The listing builds one solid part. Answer for the finished solid, in the listing's coordinates (mm). Face numbers are marked on the shaded views. A direction names the side the tool comes from. Coordinates: 2 decimals unless noted, no trailing zeros. Order: outer loops, then holes, each group sorted by start corner. A loop starts at its lowest first (then second) coordinate and runs counter-clockwise, first axis right, second up. Notation, with made-up numbers: (40, 45.25) -> (55, 45.25) arc R35 cw to (55, 78.25) -> close; hole circle Ø1 at (23.25, 71.5). An arc over 180 degrees is marked (long way). Write item = value, one per line. Start each with the question number.
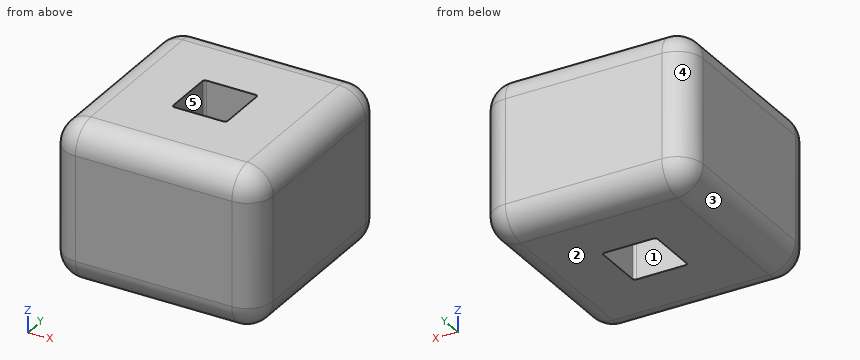
```python
from build123d import *

# Parameters (mm, degrees)
F0_W     = 400
F0_H     = 400
F0_W_2   = 104.0003
F0_H_2   = 104.0003
F1_DEPTH = 300
F2_R     = 50
F3_R     = 5


with BuildPart() as f1:
    # F0 (on Top) → F1 (new body)
    with BuildSketch(Plane.XY):
        with Locations((25.848805, -81.028401)):
            Rectangle(F0_W, F0_H)
        with Locations((25.848655, -81.028551)):
            Rectangle(F0_W_2, F0_H_2, mode=Mode.SUBTRACT)
    extrude(amount=F1_DEPTH)

    # F2
    f2_edges = [f1.edges().sort_by_distance(p)[0] for p in [
        (-174.151195, -281.028401, 150),
        (225.848805, -281.028401, 150),
        (25.848805, -281.028401, 0),
        (25.848805, -281.028401, 300),
        (225.848805, 118.971599, 150),
        (225.848805, -81.028401, 0),
        (225.848805, -81.028401, 300),
        (-174.151195, 118.971599, 150),
        (25.848805, 118.971599, 0),
        (25.848805, 118.971599, 300),
        (-174.151195, -81.028401, 0),
        (-174.151195, -81.028401, 300),
    ]]
    fillet(f2_edges, radius=F2_R)

    # F3
    f3_edges = [f1.edges().sort_by_distance(p)[0] for p in [
        (-26.151495, -29.028401, 150),
        (77.848805, -29.028401, 150),
        (77.848805, -133.028701, 150),
        (-26.151495, -133.028701, 150),
    ]]
    fillet(f3_edges, radius=F3_R)


solid = f1.part
```
Item 1: Section B-B, the plane x = 3.5 is taken. Give the vertices of the cut face in (y, z), then the cut area to 3 significant figures.
Item 2: Consider probe 1 along X at (y, z) = (-100, 196.5); probe 2 along Y at (x, z) = (15, 178.5); probe 3 along X at (y, z) = (-79.5, 285.5). Determine where each line is inside the solid, lowest interval first.
Item 3: Section A-A, the plane y = -59 is taken. Give the vertices of the cut face in (x, z), then the cut area to 3 significant figures.
Item 4: This flat-tipped pin is pushed along its axis until it touches: pin 1 (12 mm diameter, centred on y = 77, z = 256.5, fed in from +X). Where does it stop, or does it pass through?
Item 5: Section D-D, the plane z = 76 is taken. Give the vertices of the cut face in (x, y).
Item 6: For a pull along Y with two mould halves and no side action, classify the marked faces 3, 4 and 5 as pulls with the +Y half, pulls with the -Y half, needs draft (parallel to the pull), parting line crosses it, or undercut.
Item 7: Section C-C, the plane x = -116 is taken. Give the vertices of the cut face in (y, z).
Item 8: Which of the six approach directions +Z, -Z, +X, -X, +Y, -Y give full straight-line access (tool end or side, diameter ignored) to the marked faces 1 and 2?
A:
q1.outline = (-281.03, 50) arc R50 ccw to (-231.03, 0) -> (-133.03, 0) -> (-133.03, 300) -> (-231.03, 300) arc R50 ccw to (-281.03, 250) -> close; (-29.03, 0) -> (68.97, 0) arc R50 ccw to (118.97, 50) -> (118.97, 250) arc R50 ccw to (68.97, 300) -> (-29.03, 300) -> close
q1.area = 86,700 mm^2
q2.probe_1 = -174.15 to -26.15, 77.85 to 225.85
q2.probe_2 = -281.03 to -133.03, -29.03 to 118.97
q2.probe_3 = -159.36 to -26.15, 77.85 to 211.06
q3.outline = (-174.15, 50) arc R50 ccw to (-124.15, 0) -> (-26.15, 0) -> (-26.15, 300) -> (-124.15, 300) arc R50 ccw to (-174.15, 250) -> close; (77.85, 0) -> (175.85, 0) arc R50 ccw to (225.85, 50) -> (225.85, 250) arc R50 ccw to (175.85, 300) -> (77.85, 300) -> close
q3.area = 86,700 mm^2
q4.pin_1 = 225.66
q5.outline = (-174.15, -231.03) arc R50 ccw to (-124.15, -281.03) -> (175.85, -281.03) arc R50 ccw to (225.85, -231.03) -> (225.85, 68.97) arc R50 ccw to (175.85, 118.97) -> (-124.15, 118.97) arc R50 ccw to (-174.15, 68.97) -> close; hole (-26.15, -128.03) arc R5 ccw to (-21.15, -133.03) -> (72.85, -133.03) arc R5 ccw to (77.85, -128.03) -> (77.85, -34.03) arc R5 ccw to (72.85, -29.03) -> (-21.15, -29.03) arc R5 ccw to (-26.15, -34.03) -> close
q6.face_3 = needs draft
q6.face_4 = pulls with the +Y half
q6.face_5 = undercut
q7.outline = (-281.03, 50) arc R50 ccw to (-231.03, 0) -> (68.97, 0) arc R50 ccw to (118.97, 50) -> (118.97, 250) arc R50 ccw to (68.97, 300) -> (-231.03, 300) arc R50 ccw to (-281.03, 250) -> close
q8.face_1 = +Z, -Z
q8.face_2 = -Z, +X, -X, +Y, -Y
